Input: part model. Units: mm. Frame: model coordinates. A direction names the side the tool comes from. Coordinates: 2 decimals unless noted, no trailing zeros. Write each loop counter-clockwise with the first axis right and the second up, starting at its lowest first coordinate (ties: lowest second). Pieces come first, ordered by that corner, then holes.
from build123d import *

# Parameters (mm, degrees)
F1_DEPTH = 12.7
F2_W     = 14.7177
F2_H     = 9.450314
F3_DEPTH = 12.7


with BuildPart() as f1:
    # F0 (on Top) → F1 (new body)
    with BuildSketch(Plane.XY):
        Polygon((-14.7177, -9.450314), (14.7177, -9.450314), (14.7177, 9.450314), (-14.7177, 9.450314), (-14.7177, 0), align=None)
    extrude(amount=F1_DEPTH)

    # F2 (on face) → F3 (join)
    with BuildSketch(Plane.XY.offset(12.7)):
        with Locations((-7.35885, -4.725157)):
            Rectangle(F2_W, F2_H)
        with Locations((-7.35885, 4.725157)):
            Rectangle(F2_W, F2_H)
    extrude(amount=F3_DEPTH)


solid = f1.part
Item 1: Section query B-B, the plane x = 12.75. Return loops of the section in (y, z).
Item 2: Pin query (flat end, axial travel): pin 1 Ø1 at (y, z) = (0, 18.5) entering from +X; pin 2 Ø7.5 at (x, y) = (5.5, 3) entering from +Z. Return the tip coordinate at first contact, or that it passes through.
Item 3: Material intervals for line 1 (X direction, y = -6, z = 16.75); line 2 (Z direction, x = 4, y = 6), sorted ascending.
Item 4: Access query for faces 1 (the face through (14.718, 0, 6)), 2 (the face through (7, 0, 12.7)). Directions: +Z, -Z, +X, -X, +Y, -Y. A direction counts if a zero-diameter tool reaches every point of the face in a straight line with its end or side. Return the directions, or none.
Item 5: Section query C-C, the plane z = 14. Return loops of the section in (x, y), then the cut area to 3 significant figures.
Item 6: Section query A-A, the plane y = 0.5. Return loops of the section in (x, z), then the cut area to 3 significant figures.
The answers:
1. outline: (-9.45, 0) - (9.45, 0) - (9.45, 12.7) - (-9.45, 12.7) - close
2. pin 1: stops at x = 0
2. pin 2: stops at z = 12.7
3. line 1: x = -14.72 to 0
3. line 2: z = 0 to 12.7
4. face 1: +Z, -Z, +X, +Y, -Y
4. face 2: +Z, +X, +Y, -Y
5. outline: (-14.72, -9.45) - (0, -9.45) - (0, 9.45) - (-14.72, 9.45) - close
5. area: 278 mm2
6. outline: (-14.72, 0) - (14.72, 0) - (14.72, 12.7) - (0, 12.7) - (0, 25.4) - (-14.72, 25.4) - close
6. area: 561 mm2
